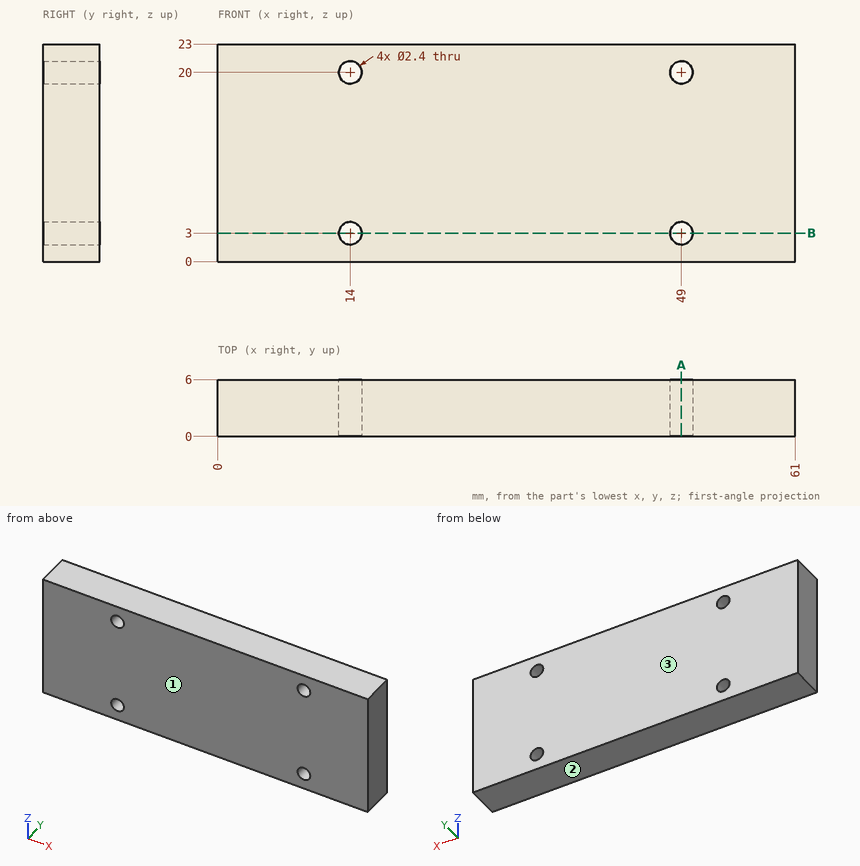
Source: three-view drawing plus pictorial views. Frame: mm from the lowest corner of the part. Give positions to 0.01 mm unless a question says otherwise; leave off trailing zeros. Order: outer loops, then holes, each group sorted by start corner. A loop starts at its lowest first (then second) coordinate and runs counter-clockwise, first axis right, second up.
1. Section A-A on x = 49. Return the cut outline in (y, z), and give its area (3 significant figures).
Derived:
outline: (0, 0) - (6, 0) - (6, 1.8) - (0, 1.8) - close; (0, 4.2) - (6, 4.2) - (6, 18.8) - (0, 18.8) - close; (0, 21.2) - (6, 21.2) - (6, 23) - (0, 23) - close
area: 109 mm2
2. Pin query (flat end, axial travel): pin 1 (1.4 mm diameter, centred on x = 14, z = 3, fed in from +Y). Return the tip coordinate at first contact, or that it passes through.
Derived:
pin 1: passes through
3. Section B-B on z = 3. Return the cut outline in (x, y), and give its area (3 significant figures).
Derived:
outline: (0, 0) - (12.8, 0) - (12.8, 6) - (0, 6) - close; (15.2, 0) - (47.8, 0) - (47.8, 6) - (15.2, 6) - close; (50.2, 0) - (61, 0) - (61, 6) - (50.2, 6) - close
area: 337 mm2
4. Mould query, pull axis Y, two halves, no side actions, for the marked faces 1, 2 and 3. Classes: released by +Y, released by -Y, zero draft, split by the parting line, or undercut.
Derived:
face 1: released by -Y
face 2: zero draft
face 3: released by +Y
5. Material intervals for L1, parallel to Z at x = 49, y = 1.85; L2, parallel to X at y = 3.25, z = 20; L3, parallel to X at y = 1, z = 4, sorted ascending.
Derived:
L1: z = 0 to 1.8, 4.2 to 18.8, 21.2 to 23
L2: x = 0 to 12.8, 15.2 to 47.8, 50.2 to 61
L3: x = 0 to 13.34, 14.66 to 48.34, 49.66 to 61
